```python
from build123d import *


with BuildPart() as part:
    # Sketch1 → Revolve1 (revolve)
    with BuildSketch(Plane.XY, mode=Mode.PRIVATE) as revolve1_sk:
        with BuildLine():
            Line((0, 4), (0, 0))
            Line((0, 0), (500, 0))
            Line((500, 0), (500, 2.5))
            Line((500, 2.5), (499.5, 3))
            Line((499.5, 3), (475.3, 3))
            ThreePointArc((475.3, 3), (475.087867966, 3.087867966), (475, 3.3))
            Line((475, 3.3), (475, 4))
            Line((475, 4), (0, 4))
        make_face()
    revolve(revolve1_sk.sketch.rotate(Axis((0, 0, 0), (1, 0, 0)), 270), axis=Axis((0, 0, 0), (1, 0, 0)))


solid = part.part
```
Could you check a few things on this model? Use its own coordinates, in mm. A direction names the side the tool comes from. Give positions to 0.01 mm unless a question says otherwise; leave off trailing zeros. Loops run counter-clockwise (first coordinate to the right, second up) from the corner with the lowest first, then second, coordinate; pieces in that order, holes last. Notation, with made-up numbers: (11, 25) - (20, 25) arc R31 ccw to (20, 60) - close; hole circle Ø6 at (-31, 34.25). An arc over 180 degrees is marked (long way). Use one line per item in the form item = value.
1. On a 3-axis mill with a long thin cutter (end or side, diameter ignored), from which of +Z, -Z, +X, -X, +Y, -Y can I reach the whole of each face in a straight line? I mean faces 1 (the face through (234.175, -3.905, 0.867)), 2 (the face through (475, 3, -2)). Say none if no direction works.
Response values:
face_1 = +X, -X
face_2 = +X
2. I want a section at A-A (x = 276.5). Please give me the cut outline in (y, z), and give its area (3 significant figures).
Response values:
outline = circle Ø8 at (0, 0)
area = 50.3 mm²
3. I need wall thicknesses on probe 1 along X at (y, z) = (1.5, 3); probe 2 along Y at (x, z) = (162, -0.5); probe 3 along Z at (x, y) = (55, 0.75). Which ranges of each line are inside material? Lowest first, please.
Response values:
probe_1 = 0 to 475
probe_2 = -3.97 to 3.97
probe_3 = -3.93 to 3.93
4. I'm going to push flat-ended pins straight in: pin 1 Ø1 at (x, z) = (224, 1) entering from +Y; pin 2 Ø1.5 at (x, y) = (269.5, -1) entering from +Z. Where does each tip first touch, or does it pass through?
Response values:
pin_1 = 3.97
pin_2 = 3.99
